Read the model definition and answer for the solid it produces. Units are mm, in the model's axes. Coordinates: 2 decimals unless noted, no trailing zeros. Write each loop counter-clockwise with the first axis right and the second up, starting at its lowest first coordinate (ties: lowest second). Pieces come first, ordered by that corner, then holes. Notation, with made-up numbers: (64, 55) - (100, 55) arc R13 ccw to (100, 64) - close; hole circle Ø3 at (-21.75, -39.5). An arc over 180 degrees is marked (long way). Return JSON: item names as keys, results as strings.
```python
from build123d import *

# Parameters (mm, degrees)
SKETCH1_R           = 175
BOSS_EXTRUDE1_DEPTH = 1.6
SKETCH2_W           = 15
SKETCH2_H           = 60
CUT_EXTRUDE1_DEPTH  = 2.6


with BuildPart() as part:
    # Sketch1 → Boss-Extrude1 (new body)
    with BuildSketch(Plane.XY):
        Circle(SKETCH1_R)
    extrude(amount=BOSS_EXTRUDE1_DEPTH)

    # Sketch2 → Cut-Extrude1 (cut, through all)
    with BuildSketch(Plane.XY.offset(1.6)):
        with Locations((-131.5, 0)):
            Rectangle(SKETCH2_W, SKETCH2_H)
        with Locations((131.5, 0)):
            Rectangle(SKETCH2_W, SKETCH2_H)
    extrude(amount=-CUT_EXTRUDE1_DEPTH, mode=Mode.SUBTRACT)


solid = part.part
```
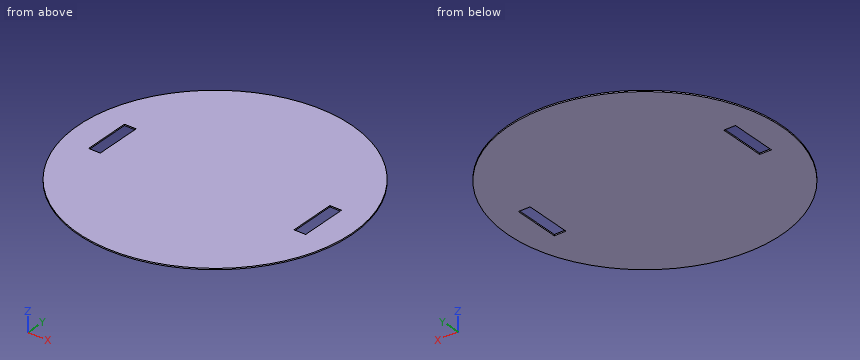
(1) A cutting plane is placed at B-B (z = 1.1). Determine the outline of the cut face in (x, y), and give its area (3 significant figures).
Answer:
{"outline": "circle Ø350 at (0, 0); hole (-139, -30) - (-124, -30) - (-124, 30) - (-139, 30) - close; hole (124, -30) - (139, -30) - (139, 30) - (124, 30) - close", "area": "94,400 mm²"}
(2) Straight lines are drawn through the part: line 1 (X direction, y = -15.5, z = 0.7); line 2 (X direction, y = 12, z = 1.05); line 3 (Y direction, x = 12, z = 0.85). For each, find the intervals that lie inside material, in ascending order. Write a range as from..to.
Answer:
{"line 1": "-174.31..-139, -124..124, 139..174.31", "line 2": "-174.59..-139, -124..124, 139..174.59", "line 3": "-174.59..174.59"}
(3) Flat-ended cylindrical pins translate along their axes: P1, Ø4, axis at x = -93, y = 8, coming from the -Z side; P2, Ø0.5, axis at x = 134.5, z = 1, coming from the -Y side; P3, Ø0.8, axis at y = 5.5, z = 1, coming from the +X side; P4, Ø0.8, axis at x = 132.5, z = 0.5, coming from the +Y side. Find the tip coordinate at first contact, or state that the pin passes through.
Answer:
{"P1": "z = 0", "P2": "y = -112.26", "P3": "x = 174.93", "P4": "y = 114.78"}
(4) A cutting plane is placed at D-D (y = -38.5). Determine the outline of the cut face in (x, z), and give its area (3 significant figures).
Answer:
{"outline": "(-170.71, 0) - (170.71, 0) - (170.71, 1.6) - (-170.71, 1.6) - close", "area": "546 mm²"}
(5) A cutting plane is placed at A-A (y = 0). Determine the outline of the cut face in (x, z).
Answer:
{"outline": "(-175, 0) - (-139, 0) - (-139, 1.6) - (-175, 1.6) - close; (-124, 0) - (124, 0) - (124, 1.6) - (-124, 1.6) - close; (139, 0) - (175, 0) - (175, 1.6) - (139, 1.6) - close"}
(6) A cutting plane is placed at C-C (x = 88). Determine the outline of the cut face in (y, z), and give its area (3 significant figures).
Answer:
{"outline": "(-151.26, 0) - (151.26, 0) - (151.26, 1.6) - (-151.26, 1.6) - close", "area": "484 mm²"}
